Design review of the part shown in the three views and the two pictorial views. Dimensions are in mm from the part's minimum x, y and z. A direction names the side the tool comes from. Round coordinates to 2 decimals unless told otherwise and drop trailing zeros. Loops run counter-clockwise (first coordinate to the right, second up) from the corner with the lowest first, then second, coordinate; pieces in that order, holes last. Notation, with made-up numbers: (-29, 61.25) -> (8, 61.25) arc R25 cw to (8, 85.25) -> close; hole circle Ø11 at (-28, -19). An arc over 180 degrees is marked (long way). Return JSON: item names as keys, results as strings. Group by question number.
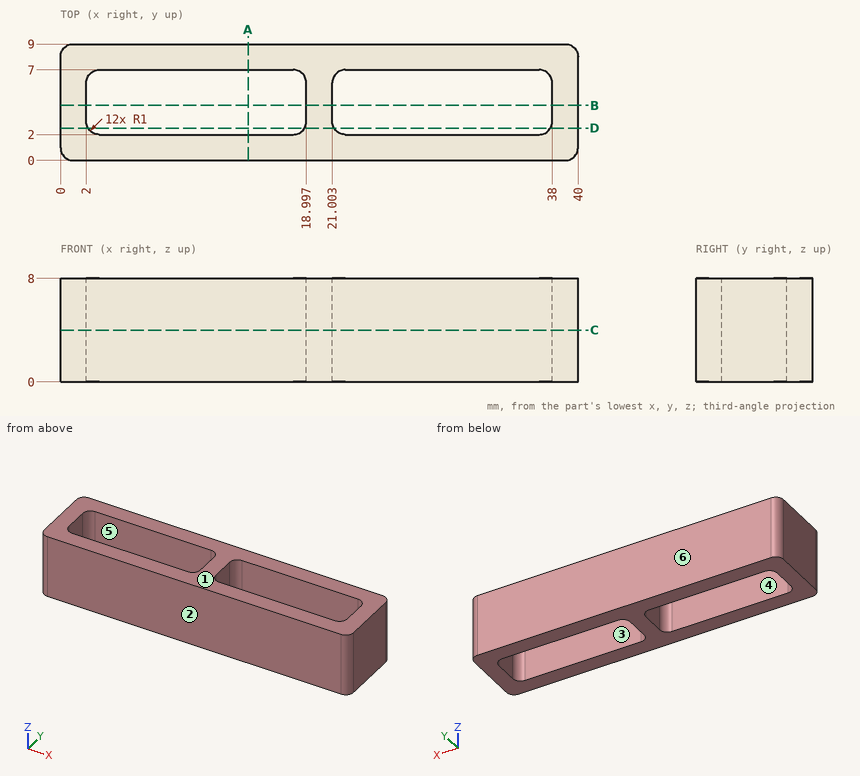
1. We need section B-B, the plane y = 4.25. Write out the cut boundary in (x, z).
2. Tool access review of the marked faces 5 and 6: name each direction out of +Z, -Z, +X, -X, +Y, -Y from which nothing blocks a thin tool from reaching the whole face with its end or side.
3. We need section D-D, the plane y = 2.5. Write out the cut boundary in (x, z).
4. Wall thickness on line 1 (Y direction, x = 26, z = 3.75); line 2 (X direction, y = 3, z = 1.5); line 3 (X direction, y = 2.25, z = 2.75): over which ranges is each line inside the solid? List them lowest first.
5. We need section A-A, the plane x = 14.5. Write out the cut boundary in (y, z), then the cut area to 3 significant figures.
6. Draft analysis for pull direction Y (two halves, no side actions). For the marked faces 1, 2, 3 and 4, state which applies: pulls with the +Y half, pulls with the -Y half, needs draft (parallel to the pull), parting line crosses it, or undercut.
7. For P1, Ø1.5, axis at x = 13.5, y = 5, coming from the -Z side, flat-tipped, find the tip position at first contact; note if it passes through.
8. We need section C-C, the plane z = 4. Write out the cut boundary in (x, y), then the cut area to 3 significant figures.
Check sheet entries:
{
 "1": {"outline": "(0, 0) -> (2, 0) -> (2, 8) -> (0, 8) -> close; (19, 0) -> (21, 0) -> (21, 8) -> (19, 8) -> close; (38, 0) -> (40, 0) -> (40, 8) -> (38, 8) -> close"},
 "2": {"face 5": "+Z, -Z", "face 6": "+Z, -Z, +X, -X, +Y"},
 "3": {"outline": "(0, 0) -> (2.13, 0) -> (2.13, 8) -> (0, 8) -> close; (18.86, 0) -> (21.14, 0) -> (21.14, 8) -> (18.86, 8) -> close; (37.87, 0) -> (40, 0) -> (40, 8) -> (37.87, 8) -> close"},
 "4": {"line 1": "y = 0 to 2, 7 to 9", "line 2": "x = 0 to 2, 19 to 21, 38 to 40", "line 3": "x = 0 to 2.34, 18.66 to 21.34, 37.66 to 40"},
 "5": {"outline": "(0, 0) -> (2, 0) -> (2, 8) -> (0, 8) -> close; (7, 0) -> (9, 0) -> (9, 8) -> (7, 8) -> close", "area": "32.0 mm²"},
 "6": {"face 1": "needs draft", "face 2": "pulls with the -Y half", "face 3": "undercut", "face 4": "undercut"},
 "7": {"P1": "passes through"},
 "8": {"outline": "(0, 1) arc R1 ccw to (1, 0) -> (39, 0) arc R1 ccw to (40, 1) -> (40, 8) arc R1 ccw to (39, 9) -> (1, 9) arc R1 ccw to (0, 8) -> close; hole (2, 3) arc R1 ccw to (3, 2) -> (18, 2) arc R1 ccw to (19, 3) -> (19, 6) arc R1 ccw to (18, 7) -> (3, 7) arc R1 ccw to (2, 6) -> close; hole (21, 3) arc R1 ccw to (22, 2) -> (37, 2) arc R1 ccw to (38, 3) -> (38, 6) arc R1 ccw to (37, 7) -> (22, 7) arc R1 ccw to (21, 6) -> close", "area": "191 mm²"}
}
